Read the model definition and answer for the solid it produces. Units are mm, in the model's axes. A direction names the side the tool comes from. Give positions to 0.01 mm unless a question says otherwise; leave off trailing zeros. Order: outer loops, then holes, each group sorted by start corner. A loop starts at its lowest first (then second) coordinate and runs counter-clockwise, first axis right, second up. Notation, with made-up numbers: (-16.75, 51.5) -> (3.25, 51.5) arc R23 cw to (3.25, 76.5) -> close; hole circle Ø11 at (-5.5, 13). An arc over 180 degrees is marked (long way). Answer as CSV lines item,"result". Start each with the question number.
1) Find section A-A (z = -1). Determine the outline of the cut face in (x, y).
2) Straight lines are drawn through the part: L1, parallel to X at y = 1.75, z = 1.5; L2, parallel to Z at x = 31, y = 0.3; L3, parallel to X at y = 2.2, z = 44. For each, find the intervals that lie inside material, in ascending order. Write a range as from..to.
3) The mould has two halves that part along X. Classify faces 1 (the face through (35, 1, 1)), 2 (the face through (0, 2, 50)), 3 (the face through (-35, 1, -1)): +X half, -X half, draft (parallel to the pull), parting line (faces both ways), or undercut.
4) Flat-ended cylindrical pins translate along their axes: pin 1 Ø0.9 at (y, z) = (1, -58) entering from -X; pin 2 Ø0.9 at (y, z) = (1, 58.5) entering from +X. Find the tip coordinate at first contact, or state that the pin passes through.
5) Find section B-B (z = 44). Determine the outline of the cut face in (x, y), and give its area (3 significant figures).
6) Find section D-D (z = -44). Determine the outline of the cut face in (x, y).
7) For faces 4 (the face through (-15, 2, 10)), 5 (the face through (-28, 1, 58)), 6 (the face through (-28, 1, -59)), 7 (the face through (28, 1, 59)), determine the directions among +Z, -Z, +X, -X, +Y, -Y from which every point of the face is accessible in a straight line to the end or side of a thin tool.
8) Find section C-C (x = 8). Determine the outline of the cut face in (y, z).
```python
from build123d import *

# Parameters (mm, degrees)
SKETCH1_R           = 1.6
BOSS_EXTRUDE1_DEPTH = 3
FILLET1_R           = 7
FILLET2_R           = 1
FILLET3_R           = 50
SKETCH2_W           = 59.626658502
SKETCH2_H           = 94.260753609
CUT_EXTRUDE1_DEPTH  = 10
FILLET4_R           = 10
SKETCH3_R           = 3.048
CUT_EXTRUDE2_DEPTH  = 10


with BuildPart() as part:
    # Sketch1 → Boss-Extrude1 (new body)
    with BuildSketch(Plane(origin=(0, 0, 0), x_dir=(1, 0, 0), z_dir=(0, 1, 0))):
        Polygon((-35, -50), (-28, -50), (-28, -132), (0, -144), (28, -132), (28, -50), (35, -50), (35, 50), (28, 50), (28, 132), (0, 144), (-28, 132), (-28, 50), (-35, 50), align=None)
        with Locations(Location((-30, 44, 0), (0, 0, 270))):
            Circle(SKETCH1_R, mode=Mode.SUBTRACT)
        with Locations(Location((30, 44, 0), (0, 0, 270))):
            Circle(SKETCH1_R, mode=Mode.SUBTRACT)
        with Locations(Location((30, -44, 0), (0, 0, 270))):
            Circle(SKETCH1_R, mode=Mode.SUBTRACT)
        with Locations(Location((-30, -44, 0), (0, 0, 270))):
            Circle(SKETCH1_R, mode=Mode.SUBTRACT)
    extrude(amount=BOSS_EXTRUDE1_DEPTH)

    # Fillet1
    fillet1_edges = [part.edges().sort_by_distance(p)[0] for p in [
        (-28, 1.5, 50),
        (28, 1.5, 50),
        (28, 1.5, -50),
        (-28, 1.5, -50),
    ]]
    fillet(fillet1_edges, radius=FILLET1_R - 0.0001)  # a hair under: the kernel refuses the full size

    # Fillet2
    fillet2_edges = [part.edges().sort_by_distance(p)[0] for p in [
        (35, 1.5, -50),
        (35, 1.5, 50),
        (-35, 1.5, 50),
        (-35, 1.5, -50),
    ]]
    fillet(fillet2_edges, radius=FILLET2_R)

    # Fillet3
    fillet3_edges = [part.edges().sort_by_distance(p)[0] for p in [
        (0, 1.5, 144),
        (0, 1.5, -144),
    ]]
    fillet(fillet3_edges, radius=FILLET3_R)

    # Sketch2 → Cut-Extrude1 (cut)
    with BuildSketch(Plane(origin=(0, 3, 0), x_dir=(1, 0, 0), z_dir=(0, 1, 0))):
        with Locations((1.813329251, 117.130376805)):
            Rectangle(SKETCH2_W, SKETCH2_H)
    cut_extrude1 = extrude(amount=-CUT_EXTRUDE1_DEPTH, mode=Mode.SUBTRACT)

    # Mirror1: Cut-Extrude1 across plane
    add(cut_extrude1.mirror(Plane.XY), mode=Mode.SUBTRACT)

    # Fillet4
    fillet4_edges = [part.edges().sort_by_distance(p)[0] for p in [
        (-28, 1.5, -70),
        (28, 1.5, -70),
        (28, 1.5, 70),
        (-28, 1.5, 70),
    ]]
    fillet(fillet4_edges, radius=FILLET4_R)

    # Sketch3 → Cut-Extrude2 (cut)
    with BuildSketch(Plane(origin=(0, 3, 0), x_dir=(1, 0, 0), z_dir=(0, 1, 0))):
        with Locations(Location((0, 50, 0), (0, 0, 270))):
            Circle(SKETCH3_R)
        with BuildLine():
            Line((15, 15), (15, -35))
            ThreePointArc((15, -35), (0, -50), (-15, -35))
            Line((-15, -35), (-15, 15))
            ThreePointArc((-15, 15), (0, 30), (15, 15))
        make_face()
    extrude(amount=-CUT_EXTRUDE2_DEPTH, mode=Mode.SUBTRACT)


solid = part.part
```
Findings below:
1,outline,"(-35, 0) -> (-15, 0) -> (-15, 3) -> (-35, 3) -> close; (15, 0) -> (35, 0) -> (35, 3) -> (15, 3) -> close"
2,L1,"-35..-15, 15..35"
2,L2,"-51.26..-45.25, -42.75..42.75, 45.25..51.26"
2,L3,"-35..-31.6, -28.4..-12, 12..28.4, 31.6..35"
3,face 1,"+X half"
3,face 2,"undercut"
3,face 3,"-X half"
4,pin 1,"x = -28"
4,pin 2,"x = 28"
5,outline,"(-35, 0) -> (-31.6, 0) -> (-31.6, 3) -> (-35, 3) -> close; (-28.4, 0) -> (-12, 0) -> (-12, 3) -> (-28.4, 3) -> close; (12, 0) -> (28.4, 0) -> (28.4, 3) -> (12, 3) -> close; (31.6, 0) -> (35, 0) -> (35, 3) -> (31.6, 3) -> close"
5,area,"119 mm²"
6,outline,"(-35, 0) -> (-31.6, 0) -> (-31.6, 3) -> (-35, 3) -> close; (-28.4, 0) -> (28.4, 0) -> (28.4, 3) -> (-28.4, 3) -> close; (31.6, 0) -> (35, 0) -> (35, 3) -> (31.6, 3) -> close"
7,face 4,"+Y, -Y"
7,face 5,"+Z, -X, +Y, -Y"
7,face 6,"-Z, -X, +Y, -Y"
7,face 7,"+Z, +X, +Y, -Y"
8,outline,"(0, -70) -> (3, -70) -> (3, -27.69) -> (0, -27.69) -> close; (0, 47.69) -> (3, 47.69) -> (3, 70) -> (0, 70) -> close"
